Can you work these out from the model? Positions are in its coordinate system, mm. A direction names the side the tool comes from. Give positions to 0.01 mm unless a question says otherwise; leave off trailing zeros. Loops run counter-clockwise (first coordinate to the right, second up) from the corner with the lowest first, then second, coordinate; pieces in that order, holes last. Notation, with made-up numbers: (33, -15) -> (75, -15) arc R15 ccw to (75, 7) -> close; hole circle Ø6 at (42, 27.25). An arc over 180 degrees is marked (long way). Return JSON: item names as keys, results as strings. Group by question number.
Q1. Suppose I cut it at A-A, the plane x = 16. Please give me the cut outline in (y, z), and give its area (3 significant figures).
Q2. Suppose I cut it at D-D, the plane x = 47. Please give me the cut outline in (y, z).
Q3. I need wall thicknesses on line 1 along Y through (x, z) = (73, -1.9); line 2 along Y through (x, z) = (42, -1.7); line 3 along X through (y, z) = (154, -1.05). Which ranges of each line are inside material? Lowest first, please. Write a range as [from, to].
Q4. Suppose I cut it at B-B, the plane y = 125. Count the separate pieces of the cut face and the enclosed holes in it, and give its area (3 significant figures).
Q5. Thinking about a two-plate mould opening in X: for faces 1 (the flat face through (2, 122, -3)), 2 (the cylindrical face through (-109.85, 96.89, -1.48)), which applies, pulls with the +X half, pulls with the -X half, needs draft (parallel to the pull), parting line crosses it, or undercut?
Q6. Which directions (+Z, -Z, +X, -X, +Y, -Y) give clear straight access to the entire face, cutting with the end or side of a thin tool? Please do faces 3 (the cylindrical face through (79.155, 145.597, -1.479)), 4 (the flat face through (2, 122, 0)).
```python
from build123d import *

# Parameters (mm, degrees)
BOSS_EXTRUDE1_DEPTH = 3


with BuildPart() as part:
    # Sketch1 → Boss-Extrude1 (new body)
    with BuildSketch(Plane.XY):
        with BuildLine():
            Line((120, 80.829037687), (-120, 80.829037687))
            add(Edge.make_bspline(
                [(-130, 92.37604307), (-130, 80.829037687), (-120, 80.829037687)],
                knots=[1.570796327, 1.570796327, 1.570796327, 3.141592654, 3.141592654, 3.141592654], degree=2, weights=[1, 0.707106781, 1]))
            Line((-130, 92.37604307), (-130, 150.111069989))
            add(Edge.make_bspline(
                [(-120, 161.658075373), (-130, 161.658075373), (-130, 150.111069989)],
                knots=[0, 0, 0, 1.570796327, 1.570796327, 1.570796327], degree=2, weights=[1, 0.707106781, 1]))
            Line((-120, 161.658075373), (120, 161.658075373))
            add(Edge.make_bspline(
                [(130, 150.111069989), (130, 161.658075373), (120, 161.658075373)],
                knots=[4.71238898, 4.71238898, 4.71238898, 6.283185307, 6.283185307, 6.283185307], degree=2, weights=[1, 0.707106781, 1]))
            Line((130, 150.111069989), (130, 92.37604307))
            add(Edge.make_bspline(
                [(120, 80.829037687), (130, 80.829037687), (130, 92.37604307)],
                knots=[3.141592654, 3.141592654, 3.141592654, 4.71238898, 4.71238898, 4.71238898], degree=2, weights=[1, 0.707106781, 1]))
        make_face()
        with BuildLine():
            Line((-102.965755224, 138.564064606), (-102.965755224, 103.923048454))
            ThreePointArc((-102.965755224, 103.923048454), (-110, 96.888803678), (-117.034244776, 103.923048454))
            Line((-117.034244776, 103.923048454), (-117.034244776, 138.564064606))
            ThreePointArc((-117.034244776, 138.564064606), (-110, 145.598309381), (-102.965755224, 138.564064606))
        make_face(mode=Mode.SUBTRACT)
        with BuildLine():
            Line((-85.534244776, 138.564064606), (-85.534244776, 103.923048454))
            ThreePointArc((-85.534244776, 103.923048454), (-78.5, 96.888803678), (-71.465755224, 103.923048454))
            Line((-71.465755224, 103.923048454), (-71.465755224, 138.564064606))
            ThreePointArc((-71.465755224, 138.564064606), (-78.5, 145.598309381), (-85.534244776, 138.564064606))
        make_face(mode=Mode.SUBTRACT)
        with BuildLine():
            Line((-54.034244776, 138.564064606), (-54.034244776, 103.923048454))
            ThreePointArc((-54.034244776, 103.923048454), (-47, 96.888803678), (-39.965755224, 103.923048454))
            Line((-39.965755224, 103.923048454), (-39.965755224, 138.564064606))
            ThreePointArc((-39.965755224, 138.564064606), (-47, 145.598309381), (-54.034244776, 138.564064606))
        make_face(mode=Mode.SUBTRACT)
        with BuildLine():
            Line((-22.534244776, 138.564064606), (-22.534244776, 103.923048454))
            ThreePointArc((-22.534244776, 103.923048454), (-15.5, 96.888803678), (-8.465755224, 103.923048454))
            Line((-8.465755224, 103.923048454), (-8.465755224, 138.564064606))
            ThreePointArc((-8.465755224, 138.564064606), (-15.5, 145.598309381), (-22.534244776, 138.564064606))
        make_face(mode=Mode.SUBTRACT)
        with BuildLine():
            Line((8.965755224, 138.564064606), (8.965755224, 103.923048454))
            ThreePointArc((8.965755224, 103.923048454), (16, 96.888803678), (23.034244776, 103.923048454))
            Line((23.034244776, 103.923048454), (23.034244776, 138.564064606))
            ThreePointArc((23.034244776, 138.564064606), (16, 145.598309381), (8.965755224, 138.564064606))
        make_face(mode=Mode.SUBTRACT)
        with BuildLine():
            Line((40.465755224, 138.564064606), (40.465755224, 103.923048454))
            ThreePointArc((40.465755224, 103.923048454), (47.5, 96.888803678), (54.534244776, 103.923048454))
            Line((54.534244776, 103.923048454), (54.534244776, 138.564064606))
            ThreePointArc((54.534244776, 138.564064606), (47.5, 145.598309381), (40.465755224, 138.564064606))
        make_face(mode=Mode.SUBTRACT)
        with BuildLine():
            Line((71.965755224, 138.564064606), (71.965755224, 103.923048454))
            ThreePointArc((71.965755224, 103.923048454), (79, 96.888803678), (86.034244776, 103.923048454))
            Line((86.034244776, 103.923048454), (86.034244776, 138.564064606))
            ThreePointArc((86.034244776, 138.564064606), (79, 145.598309381), (71.965755224, 138.564064606))
        make_face(mode=Mode.SUBTRACT)
        with BuildLine():
            Line((103.465755224, 138.564064606), (103.465755224, 103.923048454))
            ThreePointArc((103.465755224, 103.923048454), (110.5, 96.888803678), (117.534244776, 103.923048454))
            Line((117.534244776, 103.923048454), (117.534244776, 138.564064606))
            ThreePointArc((117.534244776, 138.564064606), (110.5, 145.598309381), (103.465755224, 138.564064606))
        make_face(mode=Mode.SUBTRACT)
    extrude(amount=-BOSS_EXTRUDE1_DEPTH)


solid = part.part
```
Ans:
{
 "1": {"outline": "(80.83, -3) -> (96.89, -3) -> (96.89, 0) -> (80.83, 0) -> close; (145.6, -3) -> (161.66, -3) -> (161.66, 0) -> (145.6, 0) -> close", "area": "96.4 mm^2"},
 "2": {"outline": "(80.83, -3) -> (96.91, -3) -> (96.91, 0) -> (80.83, 0) -> close; (145.58, -3) -> (161.66, -3) -> (161.66, 0) -> (145.58, 0) -> close"},
 "3": {"line 1": "y = [80.83, 100.25], [142.24, 161.66]", "line 2": "y = [80.83, 99.54], [142.95, 161.66]", "line 3": "x = [-129.42, 129.42]"},
 "4": {"separate pieces": "9", "enclosed holes": "0", "area": "442 mm^2"},
 "5": {"face 1": "needs draft", "face 2": "undercut"},
 "6": {"face 3": "+Z, -Z", "face 4": "+Z, +X, -X, +Y, -Y"}
}
